Work out the finished part from the listing and answer in its coordinate system (mm). A direction names the side the tool comes from. Round coordinates to 2 decimals unless told otherwise and drop trailing zeros. Loops run counter-clockwise (first coordinate to the right, second up) from the corner with the lowest first, then second, coordinate; pieces in that order, holes last. Notation, with made-up numbers: (41.5, 34) -> (78.5, 34) arc R9 cw to (78.5, 42) -> close; hole circle Ø2 at (73.25, -11). An arc over 180 degrees is marked (long way). Use CSV: the item, a comma, the result in double quotes. Start each with the question number.
from build123d import *

# Parameters (mm, degrees)
BASE_FLANGE2_DEPTH = 35
SKETCH12_W         = 24
SKETCH12_H         = 14
CUT_EXTRUDE1_DEPTH = 4
CUT_EXTRUDE2_REACH = 48.098
SKETCH13_R         = 2


# Sheet-metal steps are written as plain solids
with BuildPart() as part:
    # Sketch7 → Base-Flange2 (new body)
    with BuildSketch(Plane.XY):
        with BuildLine():
            Line((-24, -16), (-13, -16))
            ThreePointArc((-13, -16), (-12.292893219, -15.707106781), (-12, -15))
            Line((-12, -15), (-12, -3))
            ThreePointArc((-12, -3), (-11.121320344, -0.878679656), (-9, 0))
            Line((-9, 0), (9, 0))
            ThreePointArc((9, 0), (11.121320344, -0.878679656), (12, -3))
            Line((12, -3), (12, -15))
            ThreePointArc((12, -15), (12.292893219, -15.707106781), (13, -16))
            Line((13, -16), (24, -16))
            Line((24, -16), (24, -18))
            Line((24, -18), (13, -18))
            ThreePointArc((13, -18), (10.878679656, -17.121320344), (10, -15))
            Line((10, -15), (10, -3))
            ThreePointArc((10, -3), (9.707106781, -2.292893219), (9, -2))
            Line((9, -2), (-9, -2))
            ThreePointArc((-9, -2), (-9.707106781, -2.292893219), (-10, -3))
            Line((-10, -3), (-10, -15))
            ThreePointArc((-10, -15), (-10.878679656, -17.121320344), (-13, -18))
            Line((-13, -18), (-24, -18))
            Line((-24, -18), (-24, -16))
        make_face()
    extrude(amount=BASE_FLANGE2_DEPTH)

    # Sketch12 → Cut-Extrude1 (cut)
    with BuildSketch(Plane(origin=(0, 0, 0), x_dir=(1, 0, 0), z_dir=(0, 1, 0))):
        with Locations((0, -28)):
            Rectangle(SKETCH12_W, SKETCH12_H)
    extrude(amount=-CUT_EXTRUDE1_DEPTH, mode=Mode.SUBTRACT)

    # Sketch13 → Cut-Extrude2 (cut, up to next)
    with BuildSketch(Plane(origin=(0, 0, 0), x_dir=(1, 0, 0), z_dir=(0, 1, 0)), mode=Mode.PRIVATE) as cut_extrude2_sk1:
        with Locations(Location((18.725249298, -5, 0), (0, 0, 270))):
            Circle(SKETCH13_R)
    cut_extrude2_tool1 = extrude(cut_extrude2_sk1.sketch, amount=-CUT_EXTRUDE2_REACH, mode=Mode.PRIVATE) & part.part
    # Sketch13 → Cut-Extrude2 (cut, up to next)
    with BuildSketch(Plane(origin=(0, 0, 0), x_dir=(1, 0, 0), z_dir=(0, 1, 0)), mode=Mode.PRIVATE) as cut_extrude2_sk2:
        with Locations(Location((-19.274750702, -5, 0), (0, 0, 270))):
            Circle(SKETCH13_R)
    cut_extrude2_tool2 = extrude(cut_extrude2_sk2.sketch, amount=-CUT_EXTRUDE2_REACH, mode=Mode.PRIVATE) & part.part
    # Sketch13 → Cut-Extrude2 (cut, up to next)
    with BuildSketch(Plane(origin=(0, 0, 0), x_dir=(1, 0, 0), z_dir=(0, 1, 0)), mode=Mode.PRIVATE) as cut_extrude2_sk3:
        with Locations(Location((0, -8, 0), (0, 0, 270))):
            Circle(SKETCH13_R)
    cut_extrude2_tool3 = extrude(cut_extrude2_sk3.sketch, amount=-CUT_EXTRUDE2_REACH, mode=Mode.PRIVATE) & part.part
    # Sketch13 → Cut-Extrude2 (cut, up to next)
    with BuildSketch(Plane(origin=(0, 0, 0), x_dir=(1, 0, 0), z_dir=(0, 1, 0)), mode=Mode.PRIVATE) as cut_extrude2_sk4:
        with Locations(Location((0, -16, 0), (0, 0, 270))):
            Circle(SKETCH13_R)
    cut_extrude2_tool4 = extrude(cut_extrude2_sk4.sketch, amount=-CUT_EXTRUDE2_REACH, mode=Mode.PRIVATE) & part.part
    # Sketch13 → Cut-Extrude2 (cut, up to next)
    with BuildSketch(Plane(origin=(0, 0, 0), x_dir=(1, 0, 0), z_dir=(0, 1, 0)), mode=Mode.PRIVATE) as cut_extrude2_sk5:
        with Locations(Location((18.725249298, -30, 0), (0, 0, 270))):
            Circle(SKETCH13_R)
    cut_extrude2_tool5 = extrude(cut_extrude2_sk5.sketch, amount=-CUT_EXTRUDE2_REACH, mode=Mode.PRIVATE) & part.part
    # Sketch13 → Cut-Extrude2 (cut, up to next)
    with BuildSketch(Plane(origin=(0, 0, 0), x_dir=(1, 0, 0), z_dir=(0, 1, 0)), mode=Mode.PRIVATE) as cut_extrude2_sk6:
        with Locations(Location((-19.274750702, -30, 0), (0, 0, 270))):
            Circle(SKETCH13_R)
    cut_extrude2_tool6 = extrude(cut_extrude2_sk6.sketch, amount=-CUT_EXTRUDE2_REACH, mode=Mode.PRIVATE) & part.part
    add(cut_extrude2_tool1.solids().sort_by_distance((18.725249, 0, 5))[0], mode=Mode.SUBTRACT)
    add(cut_extrude2_tool2.solids().sort_by_distance((-19.274751, 0, 5))[0], mode=Mode.SUBTRACT)
    add(cut_extrude2_tool3.solids().sort_by_distance((0, 0, 8))[0], mode=Mode.SUBTRACT)
    add(cut_extrude2_tool4.solids().sort_by_distance((0, 0, 16))[0], mode=Mode.SUBTRACT)
    add(cut_extrude2_tool5.solids().sort_by_distance((18.725249, 0, 30))[0], mode=Mode.SUBTRACT)
    add(cut_extrude2_tool6.solids().sort_by_distance((-19.274751, 0, 30))[0], mode=Mode.SUBTRACT)


solid = part.part
Q1. For a pull along Z with two mould halves and no side action, classify faces 1 (the flat face through (12, -9, 17)), 2 (the flat face through (14.4, -16.2, 35)), 3 (the cylindrical face through (-1.774, -0.986, 16.923)) as pulls with the +Z half, pulls with the -Z half, needs draft (parallel to the pull), parting line crosses it, or undercut.
Q2. Section B-B, the plane y = -3.5 is taken. Write down the section's boundary in (x, z), and give its area (3 significant figures).
Q3. Section A-A, the plane z = 33.5 is taken. Write down the section's boundary in (x, y).
Q4. Each of these flat-tipped pins is pushed along its axis until it touches: pin 1 (6 mm diameter, centred on y = -6.5, z = 16.5, fed in from -X); pin 2 (5.5 mm diameter, centred on x = -17, z = 24, fed in from +Y); pin 3 (2 mm diameter, centred on x = -6.5, z = 16.5, fed in from -Y). Where does it stop, or does it pass through?
Q5. Which of the six approach directions +Z, -Z, +X, -X, +Y, -Y give full straight-line access (tool end or side, diameter ignored) to faces 4 (the flat face through (18, -16, 17)), 5 (the flat face through (-0.2, -1.5, 21)), 6 (the flat face through (-19, -16, 17)), 7 (the flat face through (-10, -9, 17))?
Q6. Straight lines are drawn through the part: line 1 (X direction, y = -4, z = 19); line 2 (X direction, y = -16.45, z = 5); line 3 (X direction, y = -16.95, z = 30). For each, find the intervals that lie inside material, in ascending order. Write a range as from..to.
Q7. Section C-C, the plane x = 0 is taken. Write down the section's boundary in (y, z).
Q8. Section D-D, the plane z = 5 is taken. Write down the section's boundary in (x, y).
Report:
1,face 1,"needs draft"
1,face 2,"pulls with the +Z half"
1,face 3,"undercut"
2,outline,"(-12, 0) -> (-10, 0) -> (-10, 21) -> (-12, 21) -> close; (10, 0) -> (12, 0) -> (12, 21) -> (10, 21) -> close"
2,area,"84.0 mm²"
3,outline,"(-24, -18) -> (-13, -18) arc R3 ccw to (-10, -15) -> (-10, -4) -> (-12, -4) -> (-12, -15) arc R1 cw to (-13, -16) -> (-24, -16) -> close; (10, -15) arc R3 ccw to (13, -18) -> (24, -18) -> (24, -16) -> (13, -16) arc R1 cw to (12, -15) -> (12, -4) -> (10, -4) -> close"
4,pin 1,"stops at x = -12"
4,pin 2,"stops at y = -16"
4,pin 3,"stops at y = -2"
5,face 4,"+Z, -Z, +X, +Y"
5,face 5,"+Z, +X, -X, +Y"
5,face 6,"+Z, -Z, -X, +Y"
5,face 7,"+Z, -Z, -Y"
6,line 1,"x = -12..-10, 10..12"
6,line 2,"x = -24..-21.27, -17.27..-10.37, 10.37..16.73, 20.73..24"
6,line 3,"x = -24..-21.27, -17.27..-10.72, 10.72..16.73, 20.73..24"
7,outline,"(-2, 0) -> (0, 0) -> (0, 6) -> (-2, 6) -> close; (-2, 10) -> (0, 10) -> (0, 14) -> (-2, 14) -> close; (-2, 18) -> (0, 18) -> (0, 21) -> (-2, 21) -> close"
8,outline,"(-24, -18) -> (-21.27, -18) -> (-21.27, -16) -> (-24, -16) -> close; (-17.27, -18) -> (-13, -18) arc R3 ccw to (-10, -15) -> (-10, -3) arc R1 cw to (-9, -2) -> (9, -2) arc R1 cw to (10, -3) -> (10, -15) arc R3 ccw to (13, -18) -> (16.73, -18) -> (16.73, -16) -> (13, -16) arc R1 cw to (12, -15) -> (12, -3) arc R3 ccw to (9, 0) -> (-9, 0) arc R3 ccw to (-12, -3) -> (-12, -15) arc R1 cw to (-13, -16) -> (-17.27, -16) -> close; (20.73, -18) -> (24, -18) -> (24, -16) -> (20.73, -16) -> close"
